from build123d import *

# Parameters (mm, degrees)
SKETCH_R                     = 4
PAD_DEPTH                    = 12
SKETCH001_R                  = 2.2
POCKET_DEPTH                 = 6
SKETCH002_W                  = 73
SKETCH002_H                  = 81.5
SKETCH002_W_2                = 57
SKETCH002_H_2                = 65.5
PAD001_DEPTH                 = 4
SKETCH_LINEARPATTERN_2_R     = 4
PAD_LINEARPATTERN_2_DEPTH    = 12
SKETCH001_LINEARPATTERN_2_R  = 2.2
POCKET_LINEARPATTERN_2_DEPTH = 6
LINEARPATTERN001_COUNT       = 2
LINEARPATTERN001_PITCH       = 73.5
FILLET_R                     = 3.5
FILLET001_R                  = 3.5
HOLE_D                       = 3.4
HOLE_DEPTH                   = 25
HOLE_CSINK_D                 = 6.1
HOLE_CSINK_ANGLE             = 90


with BuildPart() as part:
    # Sketch → Pad (new body)
    with BuildSketch(Plane.XY):
        Circle(SKETCH_R)
    pad = extrude(amount=PAD_DEPTH)

    # Sketch001 → Pocket (cut)
    with BuildSketch(Plane.XY.offset(12)):
        Circle(SKETCH001_R)
    pocket = extrude(amount=-POCKET_DEPTH, mode=Mode.SUBTRACT)

    # Sketch002 → Pad001 (join)
    with BuildSketch(Plane.XY):
        with Locations((32.5, 36.75)):
            Rectangle(SKETCH002_W, SKETCH002_H)
        with Locations((32.5, 36.75)):
            Rectangle(SKETCH002_W_2, SKETCH002_H_2, mode=Mode.SUBTRACT)
    extrude(amount=PAD001_DEPTH)

    # Sketch LinearPattern 2 → Pad LinearPattern 2 (add)
    with BuildSketch(Plane(origin=(65, 0, 0), x_dir=(1, 0, 0), z_dir=(0, 0, 1))):
        Circle(SKETCH_LINEARPATTERN_2_R)
    pad_linearpattern_2 = extrude(amount=PAD_LINEARPATTERN_2_DEPTH)

    # Sketch001 LinearPattern 2 → Pocket LinearPattern 2 (cut)
    with BuildSketch(Plane(origin=(65, 0, 12), x_dir=(1, 0, 0), z_dir=(0, 0, 1))):
        Circle(SKETCH001_LINEARPATTERN_2_R)
    pocket_linearpattern_2 = extrude(amount=-POCKET_LINEARPATTERN_2_DEPTH, mode=Mode.SUBTRACT)

    # LinearPattern001: Pad, Pocket, Pad LinearPattern 2, Pocket LinearPattern 2 ×2
    with Locations(*[(0, i * LINEARPATTERN001_PITCH, 0) for i in range(1, LINEARPATTERN001_COUNT)]):
        add(pad)
        add(pocket, mode=Mode.SUBTRACT)
        add(pad_linearpattern_2)
        add(pocket_linearpattern_2, mode=Mode.SUBTRACT)

    # Fillet
    fillet_edges = [part.edges().sort_by_distance(p)[0] for p in [
        (-4, -4, 2),
        (69, -4, 2),
        (69, 77.5, 2),
        (-4, 77.5, 2),
    ]]
    fillet(fillet_edges, radius=FILLET_R)

    # Fillet001
    fillet001_edges = [part.edges().sort_by_distance(p)[0] for p in [
        (61, 4, 2),
        (4, 4, 2),
        (4, 69.5, 2),
        (61, 69.5, 2),
    ]]
    fillet(fillet001_edges, radius=FILLET001_R)

    # Hole
    with Locations(Plane.XY.offset(4)):
        with Locations((0, 63.5), (65, 63.5), (65, 10), (0, 10)):
            CounterSinkHole(HOLE_D / 2, HOLE_CSINK_D / 2, depth=HOLE_DEPTH, counter_sink_angle=HOLE_CSINK_ANGLE)


solid = part.part
Source: CAD feature listing. Evaluate the final solid. Frame: model axes, mm. A direction names the side the tool comes from. Give positions to 0.01 mm unless a question says otherwise; leave off trailing zeros. Write each loop counter-clockwise with the first axis right and the second up, starting at its lowest first coordinate (ties: lowest second). Pieces come first, ordered by that corner, then holes. Notation, with made-up numbers: M -39.75,-18 L -33.75,-18 A19 ccw -33.75,12 Z; hole C 57.25,73 d11. An arc over 180 degrees is marked long. Answer as a JSON object with one key per item and string values.
Q1. Contact query for flat-ended pins moving along their axis: P1, Ø2, axis at x = 0.5, y = 0.5, coming from the +Z side; P2, Ø1.5, axis at y = 12.5, z = 6.5, coming from the -X side. Output: stop coordinate, or through.
Geometry check:
{"P1": "stops at z = 6", "P2": "passes through"}
Q2. Cut plane D-D, the plane y = 25. Return the cut outline in (x, z).
Geometry check:
{"outline": "M -4,0 L 4,0 L 4,4 L -4,4 Z; M 61,0 L 69,0 L 69,4 L 61,4 Z"}
Q3. Cut plane A-A, the plane z = 10. Return the cut outline in (x, y).
Geometry check:
{"outline": "C 0,0 d8; C 0,73.5 d8; C 65,0 d8; C 65,73.5 d8; hole C 0,0 d4.4; hole C 0,73.5 d4.4; hole C 65,0 d4.4; hole C 65,73.5 d4.4"}
Q4. Mould query, pull axis X, two halves, no side actions, for faces 1 (the face through (-2.95, 76.5, 2.03)), 2 (the face through (0, 74, 6)), 3 (the face through (32, -4, 2)). Classes: +X half, -X half, draft (parallel to the pull), parting line (faces both ways), or undercut.
Geometry check:
{"face 1": "-X half", "face 2": "undercut", "face 3": "draft"}
Q5. Cut plane B-B, the plane y = 10. Return the cut outline in (x, z).
Geometry check:
{"outline": "M -4,0 L -1.7,0 L -1.7,2.65 L -3.05,4 L -4,4 Z; M 1.7,0 L 4,0 L 4,4 L 3.05,4 L 1.7,2.65 Z; M 61,0 L 63.3,0 L 63.3,2.65 L 61.95,4 L 61,4 Z; M 66.7,0 L 69,0 L 69,4 L 68.05,4 L 66.7,2.65 Z"}
Q6. Ray query, line 1 along Y through (x, z) = (0, 7.6); line 2 along Y through (x, z) = (0, 1.9); line 3 along X through (y, z) = (10, 1.95). Return the intervals inside material, ascending.
Geometry check:
{"line 1": "y = -4 to -2.2, 2.2 to 4, 69.5 to 71.3, 75.7 to 77.5", "line 2": "y = -4 to 8.3, 11.7 to 61.8, 65.2 to 77.5", "line 3": "x = -4 to -1.7, 1.7 to 4, 61 to 63.3, 66.7 to 69"}
Q7. Access query for faces 4 (the face through (5, 68.45, 2.03)), 5 (the face through (3, 31, 4)), 6 (the face through (69, 36, 2)). Directions: +Z, -Z, +X, -X, +Y, -Y. A direction counts if a zero-diameter tool reaches every point of the face in a straight line with its end or side. Return the directions, or none.
Geometry check:
{"face 4": "+Z, -Z", "face 5": "+Z", "face 6": "+Z, -Z, +X, +Y, -Y"}
Q8. Cut plane C-C, the plane x = 48.5. Return the cut outline in (y, z).
Geometry check:
{"outline": "M -4,0 L 4,0 L 4,4 L -4,4 Z; M 69.5,0 L 77.5,0 L 77.5,4 L 69.5,4 Z"}
